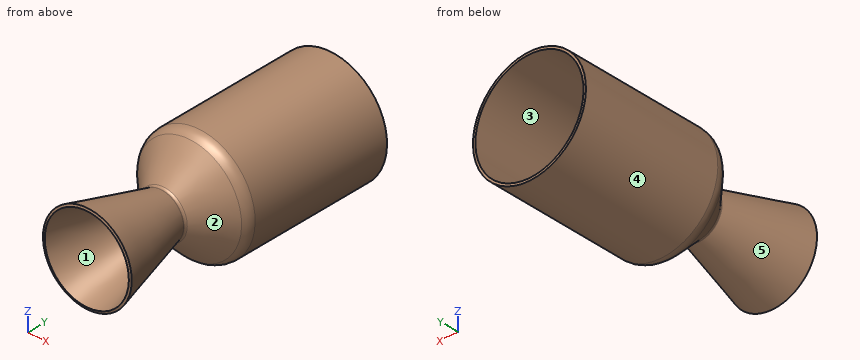
```python
from build123d import *


with BuildPart() as part:
    # Sketch1 → Revolve-Thin1 (revolve)
    with BuildSketch(Plane.XY, mode=Mode.PRIVATE) as revolve_thin1_sk:
        with BuildLine():
            Line((-57.15, 195.850768363), (-57.15, 43.450768363))
            ThreePointArc((-57.15, 43.450768363), (-56.183270063, 38.590688772), (-53.430256121, 34.470512242))
            Line((-53.430256121, 34.470512242), (-23.449871939, 4.490128061))
            ThreePointArc((-23.449871939, 4.490128061), (-22.073364969, 2.430039796), (-21.59, 0))
            ThreePointArc((-21.59, 0), (-21.622595078, -0.497304792), (-21.719822602, -0.986100562))
            Line((-21.719822602, -0.986100562), (-44.45, -85.816277477))
            Line((-44.45, -85.816277477), (-46.903451599, -85.158877102))
            Line((-46.903451599, -85.158877102), (-24.173274201, -0.328700187))
            ThreePointArc((-24.173274201, -0.328700187), (-24.140865026, -0.165768264), (-24.13, 0))
            ThreePointArc((-24.13, 0), (-24.420018981, 1.458023877), (-25.245923164, 2.694076836))
            Line((-25.245923164, 2.694076836), (-55.226307345, 32.674461018))
            ThreePointArc((-55.226307345, 32.674461018), (-58.529924075, 37.618672854), (-59.69, 43.450768363))
            Line((-59.69, 43.450768363), (-59.69, 195.850768363))
            Line((-59.69, 195.850768363), (-57.15, 195.850768363))
        make_face()
    revolve(revolve_thin1_sk.sketch.rotate(Axis((0, 0, 0), (0, 1, 0)), 270), axis=Axis((0, 0, 0), (0, 1, 0)))


solid = part.part
```
Part model, mm, in its own coordinate system. Face numbers are marked on the shaded views. A direction names the side the tool comes from. Round coordinates to 2 decimals unless told otherwise and drop trailing zeros. Write each loop counter-clockwise with the first axis right and the second up, starting at its lowest first coordinate (ties: lowest second). Pieces come first, ordered by that corner, then holes. Notation, with made-up numbers: (80.25, 48.25) -> (127.25, 48.25) arc R27 cw to (127.25, 82.25) -> close; hole circle Ø3 at (48, 69.5). An arc over 180 degrees is marked (long way). Return JSON: item names as keys, results as strings. Group by question number.
Q1. Mould opens along X. For the marked faces 1, 2 and 3 say: pulls with the +X half, pulls with the -X half, needs draft (parallel to the pull), parting line crosses it, or undercut.
Q2. Pin check, flat tips, straight feed: pin 1 (6 mm diameter, centred on y = -32.5, z = 11.5, fed in from +X); pin 2 (10 mm diameter, centred on x = 9, z = 45, fed in from +Y); pin 3 (1.5 mm diameter, centred on y = 57, z = 12, fed in from +X). Stop position of each tip, or through.
Q3. Saw through at C-C on y = 148. Write the cut outline in (x, z), plus the area to 3 significant figures.
Q4. Which spindle directions (+Z, -Z, +X, -X, +Y, -Y) get a long thin tool onto all of the face, cutting with end or side? Do the marked faces 4 and 5. Say none if no direction does.
Q5. Saw through at D-D on y = -22. Write the cut outline in (x, z).
Q6. Probe L1, parallel to X at y = 78, z = 0; L2, parallel to Z at x = 1.5, y = 126.5; L3, parallel to X at y = 79.5, z = -9. List the from-to ranges inside material, lowest first. Write a range as [from, to].
Q7. Saw through at B-B on x = 0. Write the cut outline in (y, z), plus the area to 3 significant figures.
Q8. Saw through at A-A on z = 0. Write the cut outline in (x, y), plus the area to 3 significant figures.
Answer:
{
 "1": {"face 1": "undercut", "face 2": "parting line crosses it", "face 3": "undercut"},
 "2": {"pin 1": "x = 32.02", "pin 2": "y = 31.93", "pin 3": "x = 58.62"},
 "3": {"outline": "circle Ø119.38 at (0, 0); hole circle Ø114.3 at (0, 0)", "area": "932 mm2"},
 "4": {"face 4": "+Y, -Y", "face 5": "none"},
 "5": {"outline": "circle Ø59.96 at (0, 0); hole circle Ø54.7 at (0, 0)"},
 "6": {"L1": "[-59.69, -57.15], [57.15, 59.69]", "L2": "[-59.67, -57.13], [57.13, 59.67]", "L3": "[-59.01, -56.44], [56.44, 59.01]"},
 "7": {"outline": "(-85.82, -44.45) -> (-85.16, -46.9) -> (-0.33, -24.17) arc R1.27 cw to (0, -24.13) arc R3.81 cw to (2.69, -25.25) -> (32.67, -55.23) arc R15.24 ccw to (43.45, -59.69) -> (195.85, -59.69) -> (195.85, -57.15) -> (43.45, -57.15) arc R12.7 cw to (34.47, -53.43) -> (4.49, -23.45) arc R6.35 ccw to (0, -21.59) arc R3.81 ccw to (-0.99, -21.72) -> close; (-85.82, 44.45) -> (-0.99, 21.72) arc R3.81 ccw to (0, 21.59) arc R6.35 ccw to (4.49, 23.45) -> (34.47, 53.43) arc R12.7 cw to (43.45, 57.15) -> (195.85, 57.15) -> (195.85, 59.69) -> (43.45, 59.69) arc R15.24 ccw to (32.67, 55.23) -> (2.69, 25.25) arc R3.81 cw to (0, 24.13) arc R1.27 cw to (-0.33, 24.17) -> (-85.16, 46.9) -> close", "area": "1,520 mm2"},
 "8": {"outline": "(-59.69, 43.45) arc R15.24 ccw to (-55.23, 32.67) -> (-25.25, 2.69) arc R3.81 cw to (-24.13, 0) arc R1.27 cw to (-24.17, -0.33) -> (-46.9, -85.16) -> (-44.45, -85.82) -> (-21.72, -0.99) arc R3.81 ccw to (-21.59, 0) arc R6.35 ccw to (-23.45, 4.49) -> (-53.43, 34.47) arc R12.7 cw to (-57.15, 43.45) -> (-57.15, 195.85) -> (-59.69, 195.85) -> close; (21.59, 0) arc R3.81 ccw to (21.72, -0.99) -> (44.45, -85.82) -> (46.9, -85.16) -> (24.17, -0.33) arc R1.27 cw to (24.13, 0) arc R3.81 cw to (25.25, 2.69) -> (55.23, 32.67) arc R15.24 ccw to (59.69, 43.45) -> (59.69, 195.85) -> (57.15, 195.85) -> (57.15, 43.45) arc R12.7 cw to (53.43, 34.47) -> (23.45, 4.49) arc R6.35 ccw to start", "area": "1,520 mm2"}
}
